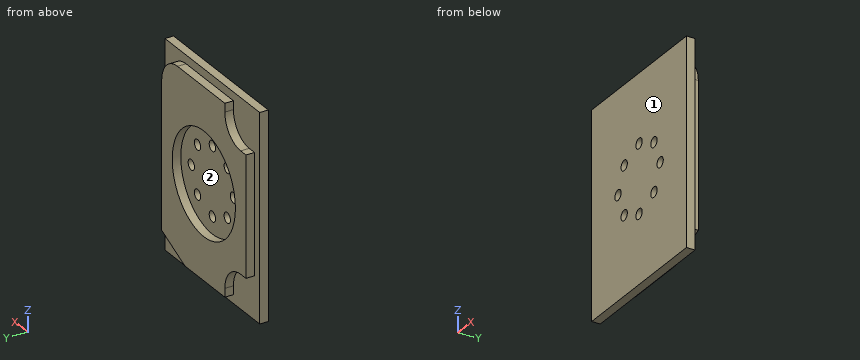
from build123d import *

# Parameters (mm, degrees)
F0_W     = 90
F0_H     = 120
F1_DEPTH = 5
F3_DEPTH = 5
F4_R     = 30
F4_R_2   = 3
F5_DEPTH = 5
F6_DEPTH = 25


with BuildPart() as f1:
    # F0 (on Front) → F1 (new body)
    with BuildSketch(Plane.XZ):
        Rectangle(F0_W, F0_H)
    extrude(amount=F1_DEPTH)

    # F2 (on face) → F3 (join)
    with BuildSketch(Plane(origin=(0, 0, 0), x_dir=(-1, 0, 0), z_dir=(0, 1, 0))):
        with BuildLine():
            Line((-40, -45), (-18, -55))
            Line((-18, -55), (20, -55))
            Line((20, -55), (20, -50))
            ThreePointArc((20, -50), (24.393398, -39.393398), (35, -35))
            Line((35, -35), (40, -35))
            Line((40, -35), (40, 35))
            Line((40, 35), (35, 35))
            ThreePointArc((35, 35), (24.393398, 39.393398), (20, 50))
            Line((20, 50), (20, 55))
            Line((20, 55), (-25, 55))
            ThreePointArc((-25, 55), (-35.606602, 50.606602), (-40, 40))
            Line((-40, 40), (-40, -45))
        make_face()
    extrude(amount=F3_DEPTH)

    # F4 (on face) → F5 (cut)
    with BuildSketch(Plane(origin=(0, 5, 0), x_dir=(-1, 0, 0), z_dir=(0, 1, 0))):
        Circle(F4_R)
        with Locations((-14.14, -14.144271)):
            Circle(F4_R_2, mode=Mode.SUBTRACT)
        with Locations((0, -20)):
            Circle(F4_R_2, mode=Mode.SUBTRACT)
        with Locations((14.14, -14.144271)):
            Circle(F4_R_2, mode=Mode.SUBTRACT)
        with Locations((-20, 0)):
            Circle(F4_R_2, mode=Mode.SUBTRACT)
        with Locations((-14.14, 14.144271)):
            Circle(F4_R_2, mode=Mode.SUBTRACT)
        with Locations((0, 20)):
            Circle(F4_R_2, mode=Mode.SUBTRACT)
        with Locations((14.14, 14.144271)):
            Circle(F4_R_2, mode=Mode.SUBTRACT)
        with Locations((20, 0)):
            Circle(F4_R_2, mode=Mode.SUBTRACT)
    extrude(amount=-F5_DEPTH, mode=Mode.SUBTRACT)

    # F4 (on face) → F6 (cut)
    with BuildSketch(Plane(origin=(0, 5, 0), x_dir=(-1, 0, 0), z_dir=(0, 1, 0))):
        with Locations((-14.14, -14.144271)):
            Circle(F4_R_2)
        with Locations((-20, 0)):
            Circle(F4_R_2)
        with Locations((-14.14, 14.144271)):
            Circle(F4_R_2)
        with Locations((0, 20)):
            Circle(F4_R_2)
        with Locations((14.14, 14.144271)):
            Circle(F4_R_2)
        with Locations((20, 0)):
            Circle(F4_R_2)
        with Locations((14.14, -14.144271)):
            Circle(F4_R_2)
        with Locations((0, -20)):
            Circle(F4_R_2)
    extrude(amount=-F6_DEPTH, mode=Mode.SUBTRACT)


solid = f1.part
Input: part model. Units: mm. Frame: model coordinates. Face numbers are marked on the shaded views. Round coordinates to 2 decimals unless told otherwise and drop trailing zeros. Write each loop counter-clockwise with the first axis right and the second up, starting at its lowest first coordinate (ties: lowest second). Pieces come first, ordered by that corner, then holes.
1) Cut plane D-D (x = 33.5). Return the cut outline in (y, z), then the cut area to 3 significant figures.
2) Ray query, L1, parallel to Z at x = 14, y = -0.5; L2, parallel to X at y = -2, z = 12; L3, parallel to Z at x = -16.5, y = -3. Return the intervals inside material, ascending.
3) Contact query for flat-ended pins moving along their axis: P1, Ø5, axis at x = 22.5, z = -12.5, coming from the +Y side; P2, Ø1.5, axis at y = 1.5, z = -52.5, coming from the -X side; P3, Ø5.5, axis at x = 0, z = 20, coming from the +Y side; P4, Ø2.5, axis at x = -36.5, y = 2.5, coming from the +Z side. Output: stop coordinate, or through.
4) Cut plane C-C (z = -20). Return the cut outline in (x, y).
5) Draft query along X for the marked faces 1 and 2. Return one class per face: pulls with the +X half, pulls with the -X half, needs draft (parallel to the pull), parting line crosses it, or undercut.
6) Cut plane A-A (y = -1.75). Count the separate pieces of the cut face and the enclosed holes in it, then the cut area to 3 significant figures.
7) Cut plane B-B (x = 14.14). Return the cut outline in (y, z).
Geometry says:
1. outline: (-5, -60) - (0, -60) - (0, -47.95) - (5, -47.95) - (5, 52.36) - (0, 52.36) - (0, 60) - (-5, 60) - close
1. area: 1,100 mm2
2. L1: z = -60 to -17.14, -11.15 to 11.15, 17.14 to 60
2. L2: x = -45 to -16.24, -12.04 to 12.04, 16.24 to 45
2. L3: z = -60 to -16, -12.29 to 12.29, 16 to 60
3. P1: stops at y = 0
3. P2: stops at x = -20
3. P3: passes through
3. P4: stops at z = 35
4. outline: (-45, -5) - (-3, -5) - (-3, 0) - (-22.36, 0) - (-22.36, 5) - (-40, 5) - (-40, 0) - (-45, 0) - close; (3, -5) - (45, -5) - (45, 0) - (40, 0) - (40, 5) - (22.36, 5) - (22.36, 0) - (3, 0) - close
5. face 1: needs draft
5. face 2: undercut
6. separate pieces: 1
6. enclosed holes: 8
6. area: 10,600 mm2
7. outline: (-5, -60) - (0, -60) - (0, -55) - (5, -55) - (5, -26.46) - (0, -26.46) - (0, -17.14) - (-5, -17.14) - close; (-5, -11.14) - (0, -11.14) - (0, 11.14) - (-5, 11.14) - close; (-5, 17.14) - (0, 17.14) - (0, 26.46) - (5, 26.46) - (5, 55) - (0, 55) - (0, 60) - (-5, 60) - close
